from build123d import *

# Parameters (mm, degrees)
F0_W     = 100
F0_H     = 100
F1_DEPTH = 150
F2_W     = 90
F2_H     = 140
F3_DEPTH = 100
F4_R     = 2.5
F5_DEPTH = 50
F6_W     = 5
F6_H     = 100
F7_DEPTH = 40


with BuildPart() as f1:
    # F0 (on Top) → F1 (new body)
    with BuildSketch(Plane.XY):
        with Locations((-4.986377, 7.071109)):
            Rectangle(F0_W, F0_H)
    extrude(amount=F1_DEPTH)

    # F2 (on face) → F3 (cut)
    with BuildSketch(Plane.XZ.offset(42.928891)):
        with Locations((-4.986377, 75)):
            Rectangle(F2_W, F2_H)
    extrude(amount=-F3_DEPTH, mode=Mode.SUBTRACT)

    # F4 (on face) → F5 (cut)
    with BuildSketch(Plane.XY.offset(150)):
        with Locations((-4.986377, 7.071109)):
            Circle(F4_R)
    extrude(amount=-F5_DEPTH, mode=Mode.SUBTRACT)

    # F6 (on face) → F7 (join)
    with BuildSketch(Plane.XY.offset(5)):
        with Locations((-22.486377, 7.071109)):
            Rectangle(F6_W, F6_H)
        with Locations((12.513623, 7.071109)):
            Rectangle(F6_W, F6_H)
    extrude(amount=F7_DEPTH)


solid = f1.part
CAD build for the part. Positions are in the model's coordinates, mm. A direction names the side the tool comes from. Give positions to 0.01 mm unless a question says otherwise; leave off trailing zeros. Loops run counter-clockwise (first coordinate to the right, second up) from the corner with the lowest first, then second, coordinate; pieces in that order, holes last. Notation, with made-up numbers: M 56.25,-35.5 L 79.25,-35.5 A17 cw 79.25,-12.5 Z; hole C 80,39 d9. An arc over 180 degrees is marked long. Answer in a Markdown table with one row per item. Add a question column.
Item 1: Probe probe 1 along X at (y, z) = (-11, 26); probe 2 along Z at (x, y) = (-48.5, 13.5); probe 3 along X at (y, z) = (42.5, 68). List the from-to ranges inside material, lowest first.
Item 2: Band-saw the part on C-C on z = 30. Give the cut face in (x, y).
Item 3: Band-saw the part on D-D on y = -26. Give the cut face in (x, z), then the cut area to 3 significant figures.
Item 4: Tool access for faces 1 (the face through (12, 8, 45)), 2 (the face through (-3.642, 9.179, 147.535)), 3 (the face through (13, 57.071, 41)): list every direction of +Z, -Z, +X, -X, +Y, -Y with a clear straight run to the whole face (end or side of a thin tool).
Item 5: Mould opens along Z. For faces 4 (the face through (-6, 19, 150)), 5 (the face through (-38, 6, 5)), 6 (the face through (-6, 8, 0)), 7 (the face through (45.014, 6, 74)) say: +Z half, -Z half, draft (parallel to the pull), parting line (faces both ways), or undercut.
Item 6: Band-saw the part on B-B on x = 8. Give the cut face in (y, z).
Item 7: Band-saw the part on A-A on z = 53. Give the cut face in (x, y), then the cut area to 3 significant figures.
Reply:
| question | item | result |
|---|---|---|
| 1 | probe 1 | x = -54.99 to -49.99, -24.99 to -19.99, 10.01 to 15.01, 40.01 to 45.01 |
| 1 | probe 2 | z = 0 to 5, 145 to 150 |
| 1 | probe 3 | x = -54.99 to -49.99, 40.01 to 45.01 |
| 2 | outline | M -54.99,-42.93 L -49.99,-42.93 L -49.99,57.07 L -54.99,57.07 Z; M -24.99,-42.93 L -19.99,-42.93 L -19.99,57.07 L -24.99,57.07 Z; M 10.01,-42.93 L 15.01,-42.93 L 15.01,57.07 L 10.01,57.07 Z; M 40.01,-42.93 L 45.01,-42.93 L 45.01,57.07 L 40.01,57.07 Z |
| 3 | outline | M -54.99,0 L 45.01,0 L 45.01,150 L -54.99,150 Z; hole M -49.99,5 L -24.99,5 L -24.99,45 L -19.99,45 L -19.99,5 L 10.01,5 L 10.01,45 L 15.01,45 L 15.01,5 L 40.01,5 L 40.01,145 L -49.99,145 Z |
| 3 | area | 2,800 mm^2 |
| 4 | face 1 | +Y, -Y |
| 4 | face 2 | +Z |
| 4 | face 3 | +Z, -Z, +X, -X, +Y |
| 5 | face 4 | +Z half |
| 5 | face 5 | undercut |
| 5 | face 6 | -Z half |
| 5 | face 7 | draft |
| 6 | outline | M -42.93,0 L 57.07,0 L 57.07,5 L -42.93,5 Z; M -42.93,145 L 57.07,145 L 57.07,150 L -42.93,150 Z |
| 7 | outline | M -54.99,-42.93 L -49.99,-42.93 L -49.99,57.07 L -54.99,57.07 Z; M 40.01,-42.93 L 45.01,-42.93 L 45.01,57.07 L 40.01,57.07 Z |
| 7 | area | 1,000 mm^2 |
